Geometry: final body of the model. Coordinates: model frame, mm. Face numbers are marked on the shaded views. Give positions to 0.01 mm unless a question says otherwise; leave off trailing zeros. Write each loop counter-clockwise with the first axis right and the second up, starting at its lowest first coordinate (ties: lowest second). Pieces come first, ordered by that corner, then holes.
```python
from build123d import *

# Parameters (mm, degrees)
SKETCH1_W           = 21
SKETCH1_H           = 51
BOSS_EXTRUDE1_DEPTH = 2
SKETCH2_W           = 8
SKETCH2_H           = 6
BOSS_EXTRUDE2_DEPTH = 2
SKETCH3_R           = 1.1
CUT_EXTRUDE1_DEPTH  = 2


with BuildPart() as part:
    # Sketch1 → Boss-Extrude1 (new body)
    with BuildSketch(Plane(origin=(0, 0, 0), x_dir=(1, 0, 0), z_dir=(0, 1, 0))):
        Rectangle(SKETCH1_W, SKETCH1_H)
    extrude(amount=BOSS_EXTRUDE1_DEPTH)

    # Sketch2 → Boss-Extrude2 (add)
    with BuildSketch(Plane(origin=(0, 2, 0), x_dir=(1, 0, 0), z_dir=(0, 1, 0))):
        with Locations((0, 22.5)):
            Rectangle(SKETCH2_W, SKETCH2_H)
    extrude(amount=BOSS_EXTRUDE2_DEPTH)

    # Sketch3 → Cut-Extrude1 (cut)
    with BuildSketch(Plane(origin=(0, 2, 0), x_dir=(1, 0, 0), z_dir=(0, 1, 0))):
        with Locations((-5.7, 23.5)):
            Circle(SKETCH3_R)
        with Locations((5.7, 23.5)):
            Circle(SKETCH3_R)
        with Locations((-5.7, -23.5)):
            Circle(SKETCH3_R)
        with Locations((5.7, -23.5)):
            Circle(SKETCH3_R)
    extrude(amount=-CUT_EXTRUDE1_DEPTH, mode=Mode.SUBTRACT)


solid = part.part
```
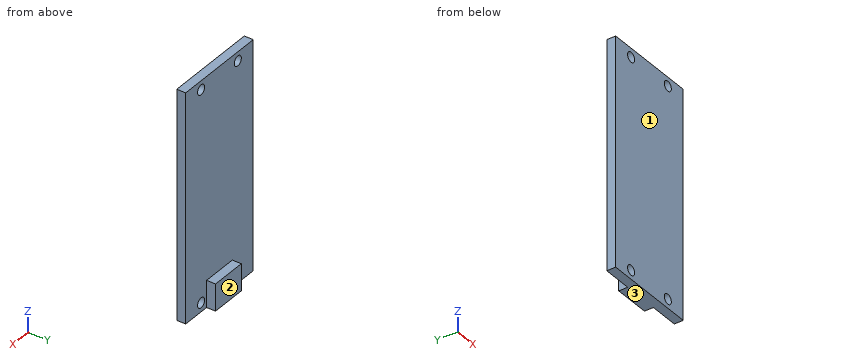
Item 1: Pull-direction query (Y, two-part tool) for the marked faces 1, 2 and 3; classes: +Y half, -Y half, draft (parallel to the pull), parting line (faces both ways), or undercut.
Found:
face 1: -Y half
face 2: +Y half
face 3: draft
Item 2: Pin query (flat end, axial travel): pin 1 Ø1.6 at (x, y) = (0.5, 3) entering from +Z; pin 2 Ø8 at (x, z) = (4, 0.5) entering from +Y; pin 3 Ø1 at (y, z) = (3, -22.5) entering from -X. Return the tip coordinate at first contact, or that it passes through.
Found:
pin 1: stops at z = -19.5
pin 2: stops at y = 2
pin 3: stops at x = -4
Item 3: Section A-A, the plane x = -5.7. Return the cut outline in (y, z), plus the area to 3 significant figures.
Found:
outline: (0, -25.5) - (2, -25.5) - (2, -24.6) - (0, -24.6) - close; (0, -22.4) - (2, -22.4) - (2, 22.4) - (0, 22.4) - close; (0, 24.6) - (2, 24.6) - (2, 25.5) - (0, 25.5) - close
area: 93.2 mm2
Item 4: Line query: L1, parallel to X at y = 0.7, z = 23.5; L2, parallel to Z at x = -5.7, y = 0.8; L3, parallel to X at y = 1.15, z = -22.5. Output: solid intervals per line, ascending.
Found:
L1: x = -10.5 to -6.8, -4.6 to 4.6, 6.8 to 10.5
L2: z = -25.5 to -24.6, -22.4 to 22.4, 24.6 to 25.5
L3: x = -10.5 to -6.16, -5.24 to 5.24, 6.16 to 10.5
Item 5: Section C-C, the plane z = 23.5. Return the cut outline in (x, y), plus the area to 3 significant figures.
Found:
outline: (-10.5, 0) - (-6.8, 0) - (-6.8, 2) - (-10.5, 2) - close; (-4.6, 0) - (4.6, 0) - (4.6, 2) - (-4.6, 2) - close; (6.8, 0) - (10.5, 0) - (10.5, 2) - (6.8, 2) - close
area: 33.2 mm2
Item 6: Section B-B, the plane z = -23.5. Return the cut outline in (x, y).
Found:
outline: (-10.5, 0) - (-6.8, 0) - (-6.8, 2) - (-10.5, 2) - close; (-4.6, 0) - (4.6, 0) - (4.6, 2) - (4, 2) - (4, 4) - (-4, 4) - (-4, 2) - (-4.6, 2) - close; (6.8, 0) - (10.5, 0) - (10.5, 2) - (6.8, 2) - close
Item 7: Section D-D, the plane x = 3.5. Return the cut outline in (y, z).
Found:
outline: (0, -25.5) - (4, -25.5) - (4, -19.5) - (2, -19.5) - (2, 25.5) - (0, 25.5) - close
